from build123d import *

# Parameters (mm, degrees)
SKETCH1_W             = 35.56
SKETCH1_H             = 20.32
BOSS_EXTRUDE1_DEPTH   = 19.05
SKETCH2_R             = 7.747
CUT_EXTRUDE1_DEPTH    = 20.05
SKETCH3_W             = 7.5451369
SKETCH3_H             = 1.27
CUT_EXTRUDE2_DEPTH    = 20.05
CUT_EXTRUDE4_DEPTH    = 2.1
F_4_CLEARANCE_HOLE1_D = 3.2639
SKETCH12_R            = 6.35
BOSS_EXTRUDE2_DEPTH   = 0.4


with BuildPart() as part:
    # Sketch1 → Boss-Extrude1 (new body)
    with BuildSketch(Plane.XY):
        with Locations((2.54, 0)):
            Rectangle(SKETCH1_W, SKETCH1_H)
    extrude(amount=BOSS_EXTRUDE1_DEPTH)

    # Sketch2 → Cut-Extrude1 (cut, through all)
    with BuildSketch(Plane.XY.offset(19.05)):
        Circle(SKETCH2_R)
    extrude(amount=-CUT_EXTRUDE1_DEPTH, mode=Mode.SUBTRACT)

    # Sketch3 → Cut-Extrude2 (cut, through all)
    with BuildSketch(Plane.XY.offset(19.05)):
        with Locations((-11.4935, 0)):
            Rectangle(SKETCH3_W, SKETCH3_H)
    extrude(amount=-CUT_EXTRUDE2_DEPTH, mode=Mode.SUBTRACT)

    # Sketch9 → Cut-Extrude4 (cut, symmetric)
    with BuildSketch(Plane(origin=(0, 0, 0), x_dir=(1, 0, 0), z_dir=(0, 1, 0))):
        with BuildLine():
            Line((11.01, -15.24), (11.01, -20.74))
            Line((11.01, -20.74), (22.01, -20.74))
            Line((22.01, -20.74), (22.01, -9.74))
            Line((22.01, -9.74), (16.51, -9.74))
            ThreePointArc((16.51, -9.74), (12.620912703, -11.350912703), (11.01, -15.24))
        make_face()
    extrude(amount=CUT_EXTRUDE4_DEPTH, both=True, mode=Mode.SUBTRACT)

    # #4 Clearance Hole1 (through all)
    with Locations(Plane(origin=(0, -10.16, 0), x_dir=(-1, 0, 0), z_dir=(0, -1, 0))):
        with Locations((11.43, -13.97), (11.43, -5.08), (-16.51, -15.24)):
            Hole(F_4_CLEARANCE_HOLE1_D / 2)

    # Sketch12 → Boss-Extrude2 (add)
    with BuildSketch(Plane(origin=(0, 0, 0), x_dir=(-1, 0, 0), z_dir=(0, 0, -1))):
        with Locations((15.24, -10.16)):
            Circle(SKETCH12_R)
        with Locations((-20.32, -10.16)):
            Circle(SKETCH12_R)
        with Locations((-20.32, 10.16)):
            Circle(SKETCH12_R)
        with Locations((15.24, 10.16)):
            Circle(SKETCH12_R)
    extrude(amount=-BOSS_EXTRUDE2_DEPTH)


solid = part.part
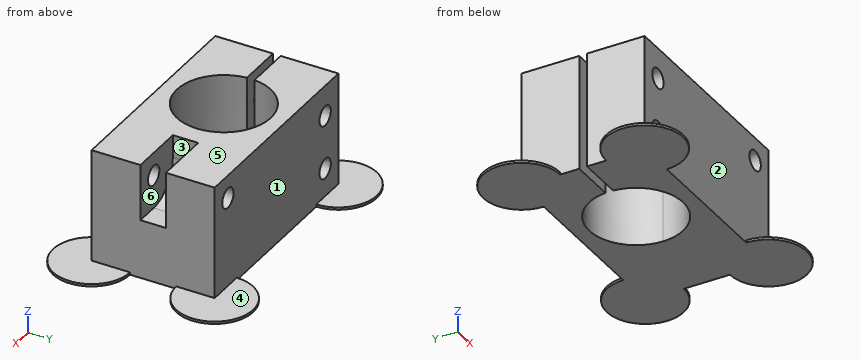
Work out the finished part from the listing and answer in its coordinate system (mm). Face numbers are marked on the shaded views. A direction names the side the tool comes from. Give positions to 0.01 mm unless a question says otherwise; leave off trailing zeros. Loops run counter-clockwise (first coordinate to the right, second up) from the corner with the lowest first, then second, coordinate; pieces in that order, holes last. Notation, with made-up numbers: (-8, -34.5) -> (15, -34.5) arc R29 cw to (15, -4.5) -> close; hole circle Ø6 at (73.5, -2.75). An arc over 180 degrees is marked (long way). Use a Markdown table: item, result. Add a question column.
1) Which of the six approach directions +Z, -Z, +X, -X, +Y, -Y give full straight-line access (tool end or side, diameter ignored) to the marked faces 5 and 6?
2) Consider line 1 along Z through (x, y) = (-11.43, -7); line 2 along Y through (x, z) = (-13.5, 15.5) (3 decimals); line 3 along X through (y, z) = (-2.25, 13.97). Determine where each line is inside the solid, lowest interval first.
3) The part is cut by section D-D, the plane z = 17.5. Determine the outline of the cut face in (x, y) (3 decimals), plus the area to 3 significant figures.
4) Each of these flat-tipped pins is pushed along its axis until it touches: P1, Ø3, axis at x = -11.43, z = 5.08, coming from the +Y side; P2, Ø4, axis at x = 21.5, y = -12, coming from the +Z side; P3, Ø2.5, axis at x = -12.5, z = 11, coming from the -Y side; P4, Ø4, axis at y = -3, z = 6, coming from the +X side. Where does it stop, or does it pass through?
5) The part is cut by section C-C, the plane x = 16. Determine the outline of the cut face in (y, z).
6) The part is cut by section B-B, the plane y = 13.5. Determine the outline of the cut face in (x, z), plus the area to 3 significant figures.
7) For a pull along Y with two mould halves and no side action, classify the marked faces 1, 2, 3 and 4 as +Y half, -Y half, draft (parallel to the pull), parting line (faces both ways), or undercut.
8) The part is cut by section A-A, the plane z = 5.08. Determine the outline of the cut face in (x, y) (3 decimals).
Reported:
| question | item | result |
|---|---|---|
| 1 | face 5 | +Z, +X, -X, +Y, -Y |
| 1 | face 6 | +Z, +X |
| 2 | line 1 | z = 0 to 3.45, 6.71 to 12.34, 15.6 to 19.05 |
| 2 | line 2 | y = -10.16 to -0.635, 0.635 to 10.16 |
| 2 | line 3 | x = -15.24 to -13.06, -9.8 to -7.41, 7.41 to 15.49, 17.53 to 20.32 |
| 3 | outline | (-15.24, -10.16) -> (20.32, -10.16) -> (20.32, -2.1) -> (11.01, -2.1) -> (11.01, 2.1) -> (20.32, 2.1) -> (20.32, 10.16) -> (-15.24, 10.16) -> (-15.24, 0.635) -> (-7.721, 0.635) arc R7.747 cw (long way) to (-7.721, -0.635) -> (-15.24, -0.635) -> close |
| 3 | area | 485 mm^2 |
| 4 | P1 | passes through |
| 4 | P2 | stops at z = 0.4 |
| 4 | P3 | stops at y = -10.16 |
| 4 | P4 | stops at x = 20.32 |
| 5 | outline | (-14.81, 0) -> (14.81, 0) -> (14.81, 0.4) -> (10.16, 0.4) -> (10.16, 13.69) -> (2.1, 13.69) -> (2.1, 9.76) -> (-2.1, 9.76) -> (-2.1, 13.69) -> (-10.16, 13.69) -> (-10.16, 0.4) -> (-14.81, 0.4) -> close; (-10.16, 16.79) -> (-2.1, 16.79) -> (-2.1, 19.05) -> (-10.16, 19.05) -> close; (2.1, 16.79) -> (10.16, 16.79) -> (10.16, 19.05) -> (2.1, 19.05) -> close |
| 6 | outline | (-20.64, 0) -> (-9.84, 0) -> (-9.84, 0.4) -> (-20.64, 0.4) -> close; (14.92, 0) -> (25.72, 0) -> (25.72, 0.4) -> (14.92, 0.4) -> close |
| 6 | area | 8.64 mm^2 |
| 7 | face 1 | +Y half |
| 7 | face 2 | -Y half |
| 7 | face 3 | undercut |
| 7 | face 4 | draft |
| 8 | outline | (-15.24, -10.16) -> (-13.062, -10.16) -> (-13.062, -0.635) -> (-15.24, -0.635) -> close; (-15.24, 0.635) -> (-13.062, 0.635) -> (-13.062, 10.16) -> (-15.24, 10.16) -> close; (-9.798, -10.16) -> (20.32, -10.16) -> (20.32, 10.16) -> (-9.798, 10.16) -> (-9.798, 0.635) -> (-7.721, 0.635) arc R7.747 cw (long way) to (-7.721, -0.635) -> (-9.798, -0.635) -> close |
